Autodesk Inventor part; units mm, degrees
ref_plane "YZ Plane" through (0, 0, 0) normal (1, 0, 0) x (0, 1, 0)
ref_plane "XZ Plane" through (0, 0, 0) normal (0, 1, 0) x (-1, 0, 0)
ref_plane "XY Plane" through (0, 0, 0) normal (0, 0, 1) x (1, 0, 0)
sketch "Sketch1" plane through (0, 0, 0) normal (0, 1, 0) x (-1, 0, 0)
  line L0 (-17.5, 48) -> (17.5, 48)
  line L1 (17.5, 48) -> (17.5, -48)
  line L2 (17.5, -48) -> (-17.5, -48)
  line L3 (-17.5, -48) -> (-17.5, 48)
  line L4 (-17.5, 48) -> (17.5, -48) construction
  line L5 (17.5, 48) -> (-17.5, -48) construction
  point P0 (0, 0)
  dimension "d0" = 96
  dimension "d1" = 35
extrude "Extrusion1" add sketch "Sketch1" along normal blind 10
fillet "Fillet1" radius 12 2 edges at (-17.5, 5, 48) (-17.5, 5, -48)
sketch "Sketch2" plane through (17.5, 0, 48) normal (0, 0, 1) x (1, 0, 0)
  line L0 (0, 10) -> (-23, 10)
  line L1 (0, 10) -> (-5, 10)
  line L2 (-5, 10) -> (-5, 6)
  line L3 (-5, 6) -> (0, 6)
  line L4 (0, 6) -> (0, 10)
  line L5 (-23, 0) -> (0, 0)
  point P0 (-17.5, 0)
  dimension "d5" = 6
  dimension "d6" = 5
extrude "Extrusion2" cut sketch "Sketch2" against normal through all
sketch "Sketch3" plane through (0, 0, 0) normal (0, 0, 1) x (1, 0, 0)
  line L0 (12.5, 10) -> (2.5, 10)
  line L1 (2.5, 10) -> (2.5, 110)
  line L2 (2.5, 110) -> (12.5, 110)
  line L3 (12.5, 110) -> (12.5, 10)
  point P0 (0, 0)
  dimension "d9" = 10
  dimension "d10" = 100
extrude "Extrusion3" add sketch "Sketch3" along normal mid plane 50
sketch "Sketch4" plane through (12.5, 6, 48) normal (1, 0, 0) x (0, 0, -1)
  line L0 (23, 104) -> (73, 104)
  circle A0 centre (48, 104) radius 15
  point P0 (48, -6)
  point P1 (63, 104)
  point P2 (33, 104)
  dimension "d13" = 30
sketch "Sketch5" plane through (12.5, 6, 48) normal (1, 0, 0) x (0, 0, -1)
  point P0 (48, -6)
extrude "Extrusion4" add sketch "Sketch4" against normal blind 50 contours A0 L0 picked at (49.773, 108.6751)
sketch "Sketch6" plane through (12.5, 6, 48) normal (1, 0, 0) x (0, 0, -1)
  line L0 (63, 104) -> (33, 104)
  circle A0 centre (48, 104) radius 15
  point P0 (48, -6)
  dimension "d16" = 30
extrude "Extrusion5" cut sketch "Sketch6" against normal blind 50
sketch "Sketch7" plane through (12.5, 6, 48) normal (1, 0, 0) x (0, 0, -1)
  arc A0 (33, 104) -> (63, 104) centre (48, 104) ccw
  circle A1 centre (48, 104) radius 15
  circle A2 centre (48, 104) radius 7.5
  point P0 (48, -6)
  dimension "d19" = 30
  dimension "d20" = 15
extrude "Extrusion6" add sketch "Sketch7" along normal blind 25
sketch "Sketch8" plane through (12.5, 6, 48) normal (-1, 0, 0) x (0, 0, 1)
  circle A0 centre (-48, 104) radius 7.5
  circle A1 centre (-48, 104) radius 15
  circle A2 centre (-48, 104) radius 7.5
  point P0 (-48, -6)
  dimension "d23" = 15
extrude "Extrusion7" add sketch "Sketch8" along normal blind 10
properties part number "gh"
Could you check a few things on this model? Use its own coordinates, in mm. A direction names the side the tool comes from. Give positions to 0.01 mm unless a question says otherwise; leave off trailing zeros. Order: outer loops, then holes, each group sorted by start corner. A loop starts at its lowest first (then second) coordinate and runs counter-clockwise, first axis right, second up.
1. Suppose I cut it at D-D (y = 80). List the corners of the cut face in (x, z) for me, plus the area to 3 significant figures.
2. Suppose I cut it at B-B (x = 15). List the corners of the cut face in (y, z) for me.
3. Will these pins go through, and if not, where does the flat tip stop? P1, Ø8, axis at x = 7, z = 22, coming from the +Y side; P2, Ø1, axis at x = 29.5, y = 104.5, coming from the -Z side; P3, Ø25, axis at y = 44, z = -6.5, coming from the -X side.
4. Suppose I cut it at A-A (z = 0). List the corners of the cut face in (x, y) for me.
5. I need wall thicknesses on L1, parallel to Y at x = 9.75, z = 0; L2, parallel to Y at x = 29, z = 0; L3, parallel to Z at x = 29, y = 110. Which ranges of each line are inside material? Lowest first, please.
6. We'd pull the mould along Y, two halves only. Please class faces 5 (the flat face through (0, 0, 1)), 6 (the flat face through (15, 6, 1)), 7 (the flat face through (7, 61, -25)): pulls with the +Y half, pulls with the -Y half, needs draft (parallel to the pull), parting line crosses it, or undercut.
7. For faces 1 (the flat face through (17.5, 3, -1)), 2 (the flat face through (7, 61, 25)), 3 (the flat face through (7, 110, -20)), 4 (the flat face through (6, 5, -48)), which set-ups out of +Z, -Z, +X, -X, +Y, -Y let a thin tool reach every point of the face, with its end or its side?
8. Suppose I cut it at C-C (x = 30.5). List the corners of the cut face in (y, z) for me.
Solved:
1. outline: (2.5, -25) - (12.5, -25) - (12.5, 25) - (2.5, 25) - close
1. area: 500 mm2
2. outline: (0, -48) - (6, -48) - (6, 48) - (0, 48) - close; circle Ø30 at (110, 0); hole circle Ø15 at (110, 0)
3. P1: stops at y = 110
3. P2: stops at z = -14.14
3. P3: stops at x = 2.5
4. outline: (-17.5, 0) - (17.5, 0) - (17.5, 6) - (12.5, 6) - (12.5, 95) - (37.5, 95) - (37.5, 102.5) - (2.5, 102.5) - (2.5, 10) - (-17.5, 10) - close; (2.5, 117.5) - (37.5, 117.5) - (37.5, 125) - (2.5, 125) - close
5. L1: y = 0 to 102.5, 117.5 to 125
5. L2: y = 95 to 102.5, 117.5 to 125
5. L3: z = -15 to -7.5, 7.5 to 15
6. face 5: pulls with the -Y half
6. face 6: undercut
6. face 7: needs draft
7. face 1: +Z, -Z, +X, -Y
7. face 2: +Z, +X, -X, +Y
7. face 3: -Z, +X, -X, +Y
7. face 4: -Z, +X, -X, +Y, -Y
8. outline: circle Ø30 at (110, 0); hole circle Ø15 at (110, 0)
